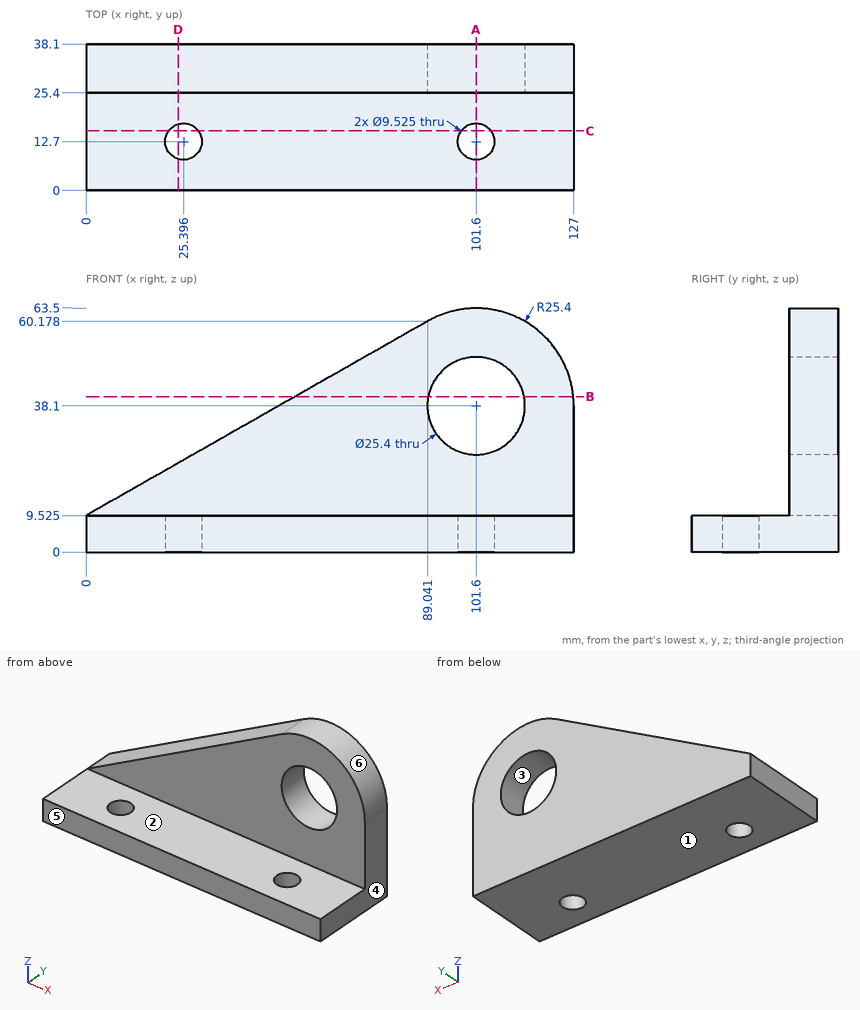
Drawing for the job (mm, zero at the part's lowest x, y, z). A direction names the side the tool comes from. Give positions to 0.01 mm unless a question says otherwise; leave off trailing zeros. Order: outer loops, then holes, each group sorted by start corner. A loop starts at its lowest first (then second) coordinate and runs counter-clockwise, first axis right, second up. Notation, with made-up numbers: (-24, 4.5) -> (14, 4.5) arc R30 ccw to (14, 36.5) -> close; hole circle Ø10 at (25, -5). An arc over 180 degrees is marked (long way). Use one line per item in the form item = value.
(1) Flat gauge pins, fed straight in: P1, Ø6, axis at x = 28, y = 23.5, coming from the -Z side; P2, Ø12.5, axis at x = 73, y = 16.5, coming from the +Z side (3 decimals); P3, Ø5.5, axis at x = 101.6, y = 12.7, coming from the -Z side. Where does each tip first touch, or does it go through?
Solution:
P1 = 0
P2 = 9.525
P3 = through
(2) Drill centre lines: line 1 (Y direction, x = 101.6, z = 3.25); line 2 (Z direction, x = 101.6, y = 29); line 3 (Z direction, x = 12, y = 21) (1 decimal). Where is each one in solid material? Low to high. Write a range as from..to.
Solution:
line_1 = 0..7.94, 17.46..38.1
line_2 = 0..25.4, 50.8..63.5
line_3 = 0..9.5
(3) Pull direction X, two halves, no side cores. Call the marked faces 3, 4, 5 and 6: +X half, -X half, draft (parallel to the pull), parting line (faces both ways), or undercut.
Solution:
face_3 = undercut
face_4 = +X half
face_5 = draft
face_6 = parting line
(4) Saw through at A-A (x = 101.6). Write the cut outline in (y, z) (1 decimal), then the cut area to 3 significant figures.
Solution:
outline = (0, 0) -> (7.9, 0) -> (7.9, 9.5) -> (0, 9.5) -> close; (17.5, 0) -> (38.1, 0) -> (38.1, 25.4) -> (25.4, 25.4) -> (25.4, 9.5) -> (17.5, 9.5) -> close; (25.4, 50.8) -> (38.1, 50.8) -> (38.1, 63.5) -> (25.4, 63.5) -> close
area = 635 mm²
(5) Saw through at C-C (y = 15.5). Count the separate pieces of the cut face and the enclosed holes in it, then the cut area to 3 significant figures.
Solution:
separate_pieces = 3
enclosed_holes = 0
area = 1,060 mm²
(6) Tool access for the marked faces 1 and 2: list every direction of +Z, -Z, +X, -X, +Y, -Y with a clear straight run to the whole face (end or side of a thin tool).
Solution:
face_1 = -Z, +X, -X, +Y, -Y
face_2 = +Z, +X, -X, -Y
(7) Saw through at B-B (z = 40.5). Write the cut outline in (x, y).
Solution:
outline = (54.45, 25.4) -> (89.13, 25.4) -> (89.13, 38.1) -> (54.45, 38.1) -> close; (114.07, 25.4) -> (126.89, 25.4) -> (126.89, 38.1) -> (114.07, 38.1) -> close
(8) Saw through at D-D (x = 24). Write the cut outline in (y, z) (1 decimal).
Solution:
outline = (0, 0) -> (8.1, 0) -> (8.1, 9.5) -> (0, 9.5) -> close; (17.3, 0) -> (38.1, 0) -> (38.1, 23.2) -> (25.4, 23.2) -> (25.4, 9.5) -> (17.3, 9.5) -> close
